The model under review builds one solid part; all positions refer to its coordinate system, in mm. A direction names the side the tool comes from. Round coordinates to 2 decimals unless told otherwise and drop trailing zeros. Order: outer loops, then holes, each group sorted by start corner. A loop starts at its lowest first (then second) coordinate and runs counter-clockwise, first axis right, second up.
Autodesk Inventor part; units mm, degrees
ref_plane "YZ Plane" through (0, 0, 0) normal (1, 0, 0) x (0, 1, 0)
ref_plane "XZ Plane" through (0, 0, 0) normal (0, 1, 0) x (-1, 0, 0)
ref_plane "XY Plane" through (0, 0, 0) normal (0, 0, 1) x (1, 0, 0)
sketch "Skizze1" plane through (0, 0, 0) normal (0, 0, 1) x (1, 0, 0)
  line L0 (-45, 2.5) -> (45, 2.5)
  line L1 (45, 2.5) -> (45, -4.5)
  line L2 (45, -4.5) -> (-45, -4.5)
  line L3 (-45, -4.5) -> (-45, 2.5)
  point P0 (0, 0)
  dimension "d0" = 7
  dimension "d1" = 90
  dimension "d2" = 45
  dimension "d3" = 2.5
extrude "Extrusion1" add sketch "Skizze1" along normal blind 20
sketch "Skizze2" plane through (0, 0, 0) normal (0, 0, -1) x (-1, 0, 0)
  line L0 (-45, 2.5) -> (45, 2.5)
  line L1 (37.5, -42.5) -> (37.5, -42.5)
  line L2 (30, -35) -> (30, 2.5)
  line L3 (30, 2.5) -> (45, 2.5)
  line L4 (45, 2.5) -> (45, -35)
  line L5 (45, 2.5) -> (45, -4.5)
  arc A0 (30, -35) -> (37.5, -42.5) centre (37.5, -35) ccw
  arc A1 (37.5, -42.5) -> (45, -35) centre (37.5, -35) ccw
  line L6 (37.5, -35) -> (37.5, -20) construction
  line L7 (40.1, -35) -> (40.1, -20)
  line L8 (34.9, -20) -> (34.9, -35)
  arc A2 (34.9, -35) -> (40.1, -35) centre (37.5, -35) ccw
  arc A3 (40.1, -20) -> (34.9, -20) centre (37.5, -20) ccw
  point P0 (0, 0)
  point P1 (37.5, -27.5)
  dimension "d8" = 45
  dimension "d9" = 7.5
  dimension "d14" = 5.2
  dimension "d15" = 15
  dimension "d16" = 4.9
  dimension "d38" = 4.9
extrude "Extrusion2" add sketch "Skizze2" against normal blind 8
fillet "Rundung2" radius 6 2 edges at (-30, -4.5, 4) (-37.5, -4.5, 8)
sketch "Skizze3" plane through (0, 0, 8) normal (0, 0, 1) x (1, 0, 0)
  line L0 (-34.9, -20) -> (-34.9, -35)
  arc A0 (-34.9, -20) -> (-40.1, -20) centre (-37.5, -20) ccw
  line L1 (-40.1, -35) -> (-40.1, -20)
  arc A1 (-40.1, -35) -> (-34.9, -35) centre (-37.5, -35) ccw
  arc A2 (-33, -20) -> (-42, -20) centre (-37.5, -20) ccw
  line L2 (-33, -20) -> (-33, -35)
  arc A3 (-42, -35) -> (-33, -35) centre (-37.5, -35) ccw
  line L3 (-42, -35) -> (-42, -20)
  point P0 (0, 0)
  dimension "d20" = 9
extrude "Extrusion3" cut sketch "Skizze3" along normal blind 5 and the other way blind 5
mirror "Spiegeln1" about plane through (0, 0, 0) normal (1, 0, 0) of "Extrusion2", "Rundung2", "Extrusion3"
sketch "Skizze4" plane through (-24, -4.5, 0) normal (0, -1, 0) x (1, 0, 0)
  line L0 (6, 14) -> (6, 6) construction
  line L1 (3.4, 14) -> (3.4, 6)
  line L2 (8.6, 6) -> (8.6, 14)
  arc A0 (8.6, 14) -> (3.4, 14) centre (6, 14) ccw
  arc A1 (3.4, 6) -> (8.6, 6) centre (6, 6) ccw
  line L3 (0, 0) -> (48, 0)
  line L4 (-21, 20) -> (69, 20)
  point P0 (24, 0)
  point P1 (6, 10)
  point P2 (52, 0)
  point P3 (69, 0)
  point P4 (-15, 20)
  dimension "d26" = 5.2
  dimension "d27" = 8
  dimension "d29" = 6
  dimension "d30" = 18
  dimension "d39" = 6
extrude "Extrusion4" cut sketch "Skizze4" against normal up to surface (7 mm away)
sketch "Skizze5" plane through (-24, -4.5, 0) normal (0, -1, 0) x (1, 0, 0)
  arc A0 (8.6, 14) -> (3.4, 14) centre (6, 14) ccw
  line L0 (3.4, 6) -> (3.4, 14)
  line L1 (8.6, 14) -> (8.6, 6)
  arc A1 (3.4, 6) -> (8.6, 6) centre (6, 6) ccw
  arc A2 (10.3, 14) -> (1.7, 14) centre (6, 14) ccw
  line L2 (10.3, 14) -> (10.3, 6)
  arc A3 (1.7, 6) -> (10.3, 6) centre (6, 6) ccw
  line L3 (1.7, 6) -> (1.7, 14)
  point P0 (24, 0)
  dimension "d33" = 8.6
extrude "Extrusion5" cut sketch "Skizze5" against normal blind 5
mirror "Spiegeln2" about plane through (0, 0, 0) normal (1, 0, 0) of "Extrusion4", "Extrusion5"
fillet "Rundung7" radius 6 2 edges at (-45, -1, 20) (45, -1, 20)
properties part number "103.007.01_Einstellwinkel" material "Aluminium 6061"
(1) For faces 4 (the cylindrical face through (-17.9, -2, 18.3)), 5 (the cylindrical face through (28.196, -6.211, 5.346)), 6 (the cylindrical face through (-17.9, 1.5, 16.6)), 7 (the flat face through (1, -4.5, 12)), list the 3-axis set-ups (+Z, -Z, +X, -X, +Y, -Y) from which the entire face can be reached by the end or side of a thin tool; tool diameter is ignored.
Data:
face 4: -Y
face 5: +Z, -Z, -Y
face 6: +Y, -Y
face 7: +Z, -Y
(2) Insertion check: pin 1 (2 mm diameter, centred on x = -10, z = 17, fed in from -Y); pin 2 (6 mm diameter, centred on y = -7.5, z = 10.5, fed in from -X); pin 3 (7 mm diameter, centred on x = 18, z = 9, fed in from -Y); pin 4 (4.5 mm diameter, centred on x = -34.5, y = -28, fed in from +Z). Each pin has a flat end and moves straight along its axis. Give the tip position at first contact, or say it passes through.
Data:
pin 1: stops at y = -4.5
pin 2: stops at x = -45
pin 3: stops at y = 0.5
pin 4: stops at z = 8
(3) Consider section D-D (z = 11). Write out the cut boundary in (x, y).
Data:
outline: (-45, -5.3) - (-27, -5.3) arc R6 cw to (-24, -4.5) - (-22.3, -4.5) - (-22.3, 0.5) - (-20.6, 0.5) - (-20.6, 2.5) - (-45, 2.5) - close; (-15.4, 0.5) - (-13.7, 0.5) - (-13.7, -4.5) - (13.7, -4.5) - (13.7, 0.5) - (15.4, 0.5) - (15.4, 2.5) - (-15.4, 2.5) - close; (20.6, 0.5) - (22.3, 0.5) - (22.3, -4.5) - (24, -4.5) arc R6 cw to (27, -5.3) - (45, -5.3) - (45, 2.5) - (20.6, 2.5) - close
(4) To check wall thickness, follow probe 1 along X at (y, z) = (-21, 7.75); probe 2 along X at (y, z) = (-1, 9.25); probe 3 along X at (y, z) = (-29, 2). State the ranges of each line that lie inside material, in increasing order.
Data:
probe 1: x = -45 to -42, -33 to -30, 30 to 33, 42 to 45
probe 2: x = -45 to -22.3, -13.7 to 13.7, 22.3 to 45
probe 3: x = -45 to -40.1, -34.9 to -30, 30 to 34.9, 40.1 to 45
(5) Draft analysis for pull direction Z (two halves, no side actions). For faces 1 (the flat face through (22.3, -2, 10)), 2 (the flat face through (32.6, -22.7, 8)), 3 (the flat face through (34.9, -28, 1)), state which applies: pulls with the +Z half, pulls with the -Z half, needs draft (parallel to the pull), parting line crosses it, or undercut.
Data:
face 1: undercut
face 2: pulls with the +Z half
face 3: needs draft
(6) Consider section A-A (x = -18). Write out the cut boundary in (y, z), and give its area (3 significant figures).
Data:
outline: (-4.5, 0) - (2.5, 0) - (2.5, 3.4) - (0.5, 3.4) - (0.5, 1.7) - (-4.5, 1.7) - close; (-4.5, 18.3) - (0.5, 18.3) - (0.5, 16.6) - (2.5, 16.6) - (2.5, 20) - (-4.5, 20) - close
area: 30.6 mm2
(7) Consider section B-B (y = -13). Write out the cut boundary in (x, z).
Data:
outline: (-45, 0) - (-30, 0) - (-30, 8) - (-45, 8) - close; (30, 0) - (45, 0) - (45, 8) - (30, 8) - close
(8) Consider section C-C (y = -33.5). Write out the cut boundary in (x, z).
Data:
outline: (-45, 0) - (-40.1, 0) - (-40.1, 3) - (-42, 3) - (-42, 8) - (-45, 8) - close; (-34.9, 0) - (-30, 0) - (-30, 8) - (-33, 8) - (-33, 3) - (-34.9, 3) - close; (30, 0) - (34.9, 0) - (34.9, 3) - (33, 3) - (33, 8) - (30, 8) - close; (40.1, 0) - (45, 0) - (45, 8) - (42, 8) - (42, 3) - (40.1, 3) - close
